For this review, take the finished solid that the model builds, in its own axes (mm). A direction names the side the tool comes from. Round coordinates to 2 decimals unless told otherwise and drop trailing zeros. Order: outer loops, then holes, each group sorted by start corner. A loop starts at its lowest first (then second) coordinate and runs counter-clockwise, first axis right, second up. Notation, with made-up numbers: (-16, 47) - (27, 47) arc R32 ccw to (27, 84) - close; hole circle Ø2 at (-23.5, 40.25). An arc over 180 degrees is marked (long way). One line per question, with ' | ' between items.
```python
from build123d import *

# Parameters (mm, degrees)
F0_R     = 11
F2_DEPTH = 6.2
F0_W     = 4.7
F0_H     = 6
F3_DEPTH = 4.7
F4_COUNT = 6
F1_W     = 0.3503125627
F1_H     = 4.9452893436
F5_DEPTH = 25.4
F6_R     = 0.762


with BuildPart() as f2:
    # F0 (on Top) → F2 (new body)
    with BuildSketch(Plane.XY):
        with BuildLine():
            ThreePointArc((-3.5, 12.5199840255), (-7.8581168228, -10.3561575886), (13, 0))
            ThreePointArc((13, 0), (10.3561575886, 7.8581168228), (3.5, 12.5199840255))
            ThreePointArc((3.5, 12.5199840255), (0, 13), (-3.5, 12.5199840255))
        make_face()
        Circle(F0_R, mode=Mode.SUBTRACT)
    extrude(amount=F2_DEPTH)

    # F0 (on Top) → F3 (join)
    with BuildSketch(Plane.XY):
        with BuildLine():
            ThreePointArc((-3.5, 12.5199840255), (0, 13), (3.5, 12.5199840255))
            Line((3.5, 12.5199840255), (3.5, 29.5199840255))
            Line((3.5, 29.5199840255), (2.35, 29.5199840255))
            Line((2.35, 29.5199840255), (-2.35, 29.5199840255))
            Line((-2.35, 29.5199840255), (-3.5, 29.5199840255))
            Line((-3.5, 29.5199840255), (-3.5, 12.5199840255))
        make_face()
        with BuildLine():
            Line((1.5, 24.2727840255), (1.5, 14.7699840255))
            Line((1.5, 14.7699840255), (1.4972, 14.7699840255))
            ThreePointArc((1.4972, 14.7699840255), (-0.6221404446, 15.647843581), (-1.5, 17.7671840255))
            Line((-1.5, 17.7671840255), (-1.5, 27.2699840255))
            Line((-1.5, 27.2699840255), (-1.4972, 27.2699840255))
            ThreePointArc((-1.4972, 27.2699840255), (0.6221404446, 26.3921244701), (1.5, 24.2727840255))
        make_face(mode=Mode.SUBTRACT)
        with Locations((0, 32.5199840255)):
            Rectangle(F0_W, F0_H)
    extrude(amount=F3_DEPTH)

    # F4: F2 ×6 about axis
    f4_axis = Axis((0, 0, 0), (0, 0, 1))


with BuildPart() as f2_1:
    add(f2.part)
    for i in range(1, F4_COUNT):
        add(f2.part.rotate(f4_axis, i * 360 / F4_COUNT))

    # F1 (on Top) → F5 (cut)
    with BuildSketch(Plane.XY):
        with Locations((-0.128307729, 13.028617017)):
            Rectangle(F1_W, F1_H)
    extrude(amount=F5_DEPTH, mode=Mode.SUBTRACT)

    # F6
    f6_edges = [f2_1.edges().sort_by_distance(p)[0] for p in [
        (-26.988132, -18.295152, 4.7),
        (-29.338132, -14.224832, 4.7),
        (-26.988132, -18.295152, 0),
        (-29.338132, -14.224832, 0),
        (-2.35, -32.519984, 0),
        (-2.35, -32.519984, 4.7),
        (2.35, -32.519984, 4.7),
        (2.35, -32.519984, 0),
        (26.988132, -18.295152, 4.7),
        (26.988132, -18.295152, 0),
        (29.338132, -14.224832, 4.7),
        (29.338132, -14.224832, 0),
        (29.338132, 14.224832, 4.7),
        (29.338132, 14.224832, 0),
        (26.988132, 18.295152, 4.7),
        (26.988132, 18.295152, 0),
        (2.35, 32.519984, 4.7),
        (2.35, 32.519984, 0),
        (-2.35, 32.519984, 4.7),
        (-2.35, 32.519984, 0),
        (-26.988132, 18.295152, 4.7),
        (-26.988132, 18.295152, 0),
        (-29.338132, 14.224832, 4.7),
        (-29.338132, 14.224832, 0),
    ]]
    fillet(f6_edges, radius=F6_R)


solid = f2_1.part
```
(1) Mouldability with a two-part tool opening along Y and no side actions: class faces 6 (the flat face through (-27, -18.3, 2.3)), 7 (the flat face through (18.694, 12.525, 2.317)), 8 (the flat face through (-20, 9, 4.7)), 9 (the cylindrical face through (27.14, 18.12, 0.22)) as released by +Y, released by -Y, zero draft, split by the parting line, or undercut.
Output values:
face 6: released by -Y | face 7: undercut | face 8: zero draft | face 9: released by +Y
(2) We need section C-C on x = -17. State the section outline as (y, z) points, plus the area to 3 significant figures.
Output values:
outline: (-13.86, 0) - (-11.55, 0) - (-11.55, 4.7) - (-13.86, 4.7) - close; (-8.08, 0) - (-5.77, 0) - (-5.77, 4.7) - (-8.08, 4.7) - close; (5.77, 0) - (8.08, 0) - (8.08, 4.7) - (5.77, 4.7) - close; (11.55, 0) - (13.86, 0) - (13.86, 4.7) - (11.55, 4.7) - close | area: 43.4 mm^2
(3) We need section D-D on y = 26. State the section outline as (x, z) points.
Output values:
outline: (-3.5, 0) - (-1.5, 0) - (-1.5, 4.7) - (-3.5, 4.7) - close; (0.95, 0) - (3.5, 0) - (3.5, 4.7) - (0.95, 4.7) - close
(4) Insertion check: pin 1 (1.6 mm diameter, centred on y = 32, z = 2, fed in from -X); pin 2 (2.5 mm diameter, centred on y = -20, z = 2.5, fed in from +X); pin 3 (17.5 mm diameter, centred on x = 0, y = 0, fed in from +Z); pin 4 (1 mm diameter, centred on y = -33.5, z = 3, fed in from +X). Each pin has a flat end and moves straight along its axis. Give the tip position at first contact, or say it passes through.
Output values:
pin 1: x = -2.35 | pin 2: x = 30.19 | pin 3: through | pin 4: x = 2.35
(5) We need section B-B on x = -10. State the section outline as (y, z) points.
Output values:
outline: (-9.81, 0) - (-4.58, 0) - (-4.58, 6.2) - (-8.31, 6.2) - (-8.31, 4.7) - (-9.81, 4.7) - close; (4.58, 0) - (9.81, 0) - (9.81, 4.7) - (8.31, 4.7) - (8.31, 6.2) - (4.58, 6.2) - close
(6) For probe 1 along X at (y, z) = (21, 3.5); probe 2 along Y at (x, z) = (0, 1.5); probe 3 along Y at (x, z) = (13.5, 0.5), list the stretches that pass through material, from the lowest coordinate up. Write a range as [from, to].
Output values:
probe 1: [-3.5, -1.5], [1.5, 3.5] | probe 2: [-35.52, -26.87], [-15.17, -11], [26.87, 35.52] | probe 3: [-11.84, -9.53], [-7.41, -3.75], [3.75, 6.16], [9.01, 11.84]
(7) For faces 1 (the flat face through (29.302, -14.204, 2.328)), 2 (the cylindrical face through (-29.26, -14.44, 0.22)), 3 (the flat face through (-29.302, 14.204, 2.328)), 4 (the cylindrical face through (-27.14, -18.12, 0.22)), 5 (the cylindrical face through (-1.175, 16.411, 2.317)), list the 3-axis set-ups (+Z, -Z, +X, -X, +Y, -Y) from which the entire face can be reached by the end or side of a thin tool; tool diameter is ignored.
Output values:
face 1: +Z, -Z, +X | face 2: -Z, -X | face 3: +Z, -Z, -X | face 4: -Z, -Y | face 5: +Z, -Z
(8) We need section A-A on y = 2. State the section outline as (x, z) points.
Output values:
outline: (-12.85, 0) - (-10.82, 0) - (-10.82, 6.2) - (-12.85, 6.2) - close; (10.82, 0) - (12.85, 0) - (12.85, 6.2) - (10.82, 6.2) - close
